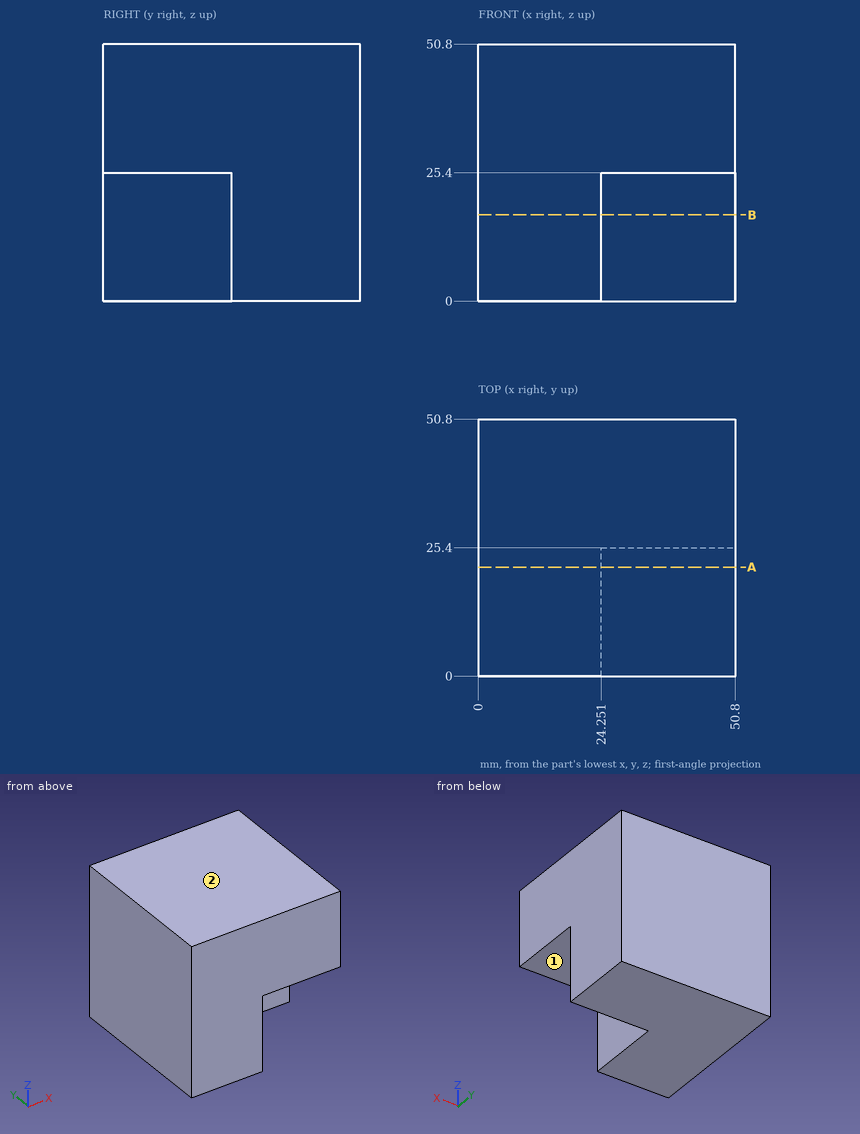
Input: dimensioned drawing with shaded views. Units: mm. Origin: part minimum x, y, z. A direction names the side the tool comes from. Coordinates: 2 decimals unless noted, no trailing zeros. Order: outer loops, then holes, each group sorted by start corner. A loop starts at its lowest first (then second) coordinate and runs counter-clockwise, first axis right, second up. Notation, with made-up numbers: (-19.75, 61) -> (-0.75, 61) arc R33 cw to (-0.75, 93) -> close; hole circle Ø2 at (28.25, 36). An arc over 180 degrees is marked (long way). Answer in a Markdown table with one row per item.
Item 1: Ray query, L1, parallel to Z at x = 44.5, y = 8.5; L2, parallel to X at y = 21, z = 11. Return the intervals inside material, ascending.
Return value:
| item | result |
|---|---|
| L1 | z = 25.4 to 50.8 |
| L2 | x = 0 to 24.25 |
Item 2: Access query for the marked faces 1 and 2. Directions: +Z, -Z, +X, -X, +Y, -Y. A direction counts if a zero-diameter tool reaches every point of the face in a straight line with its end or side. Return the directions, or none.
Return value:
| item | result |
|---|---|
| face 1 | -Z, +X, -Y |
| face 2 | +Z, +X, -X, +Y, -Y |
Item 3: Section A-A on y = 21.5. Output: boundary loops of the cut face in (x, z), plus the area to 3 significant figures.
Return value:
| item | result |
|---|---|
| outline | (0, 0) -> (24.25, 0) -> (24.25, 25.4) -> (50.8, 25.4) -> (50.8, 50.8) -> (0, 50.8) -> close |
| area | 1,910 mm² |
Item 4: Contact query for a flat-ended pin moving along its axis: P1, Ø3, axis at x = 44.5, z = 19.5, coming from the -Y side. Output: stop coordinate, or through.
Return value:
| item | result |
|---|---|
| P1 | stops at y = 25.4 |
